Autodesk Inventor part; units mm, degrees
ref_plane "YZ Plane" through (0, 0, 0) normal (1, 0, 0) x (0, 1, 0)
ref_plane "XZ Plane" through (0, 0, 0) normal (0, 1, 0) x (-1, 0, 0)
ref_plane "XY Plane" through (0, 0, 0) normal (0, 0, 1) x (1, 0, 0)
sketch "Sketch1" plane through (0, 0, 0) normal (0, 0, 1) x (1, 0, 0)
  line L0 (-22, 35) -> (22, 35)
  line L1 (22, 35) -> (22, -35)
  line L2 (22, -35) -> (-22, -35)
  line L3 (-25, -38) -> (25, -38)
  line L4 (25, -38) -> (25, 38)
  line L5 (25, 38) -> (-25, 38)
  line L6 (-25, 38) -> (-25, -38)
  line L7 (-22, -6.5359) -> (-22, 6.5359)
  arc A0 (-22, -6.5359) -> (-22, -13.4641) centre (-20, -10) ccw
  arc A1 (-22, 13.4641) -> (-22, 6.5359) centre (-20, 10) ccw
  line L8 (-22, 13.4641) -> (-22, 35)
  line L9 (-22, -35) -> (-22, -13.4641)
  point P0 (0, 0)
extrude "Extrusion1" add sketch "Sketch1" along normal blind 2 contours L0 L1 L2 L9 A0 L7 A1 L8 | L6 L5 L4 L3
sketch "Sketch2" plane through (-25, -38, 0) normal (0, -1, 0) x (1, 0, 0)
  line L0 (50, 0) -> (103.092, -17) construction
  line L1 (43.7539, 2) -> (50, 0)
  line L2 (0, 2) -> (50, 2) construction
  line L3 (50, 0) -> (50, 2)
  line L4 (43.7539, 2) -> (50, 2)
  line L5 (50, 2) -> (50, 0)
  point P0 (25, 0)
extrude "Extrusion2" cut sketch "Sketch2" against normal through all
sketch "Sketch3" plane through (0, 0, 0) normal (0, 0, -1) x (-1, 0, 0)
  line L0 (-22, -35) -> (22, -35)
  line L1 (22, 35) -> (-22, 35)
  line L2 (-22, 35) -> (-22, -35)
  line L3 (22, -35) -> (22, -13.4641)
  line L4 (22, 13.4641) -> (22, 35)
  line L5 (-21.5, -34.5) -> (21.5, -34.5)
  line L6 (21.5, -34.5) -> (21.5, -32.5)
  line L7 (21.5, -32.5) -> (-21.5, -32.5)
  line L8 (-21.5, -32.5) -> (-21.5, -34.5)
  line L9 (-21.5, 32.5) -> (21.5, 32.5)
  line L10 (21.5, 32.5) -> (21.5, 34.5)
  line L11 (21.5, 34.5) -> (-21.5, 34.5)
  line L12 (-21.5, 34.5) -> (-21.5, 32.5)
  point P0 (0, 0)
  dimension "d4" = 0.5
  dimension "d5" = 0.5
  dimension "d6" = 0.5
  dimension "d8" = 0.5
  dimension "d9" = 2
  dimension "d10" = 2
extrude "Extrusion3" add sketch "Sketch3" along normal blind 10
equation "\"d5\" = d4"
equation "\"d6\" = d4"
equation "\"d8\" = d4"
equation "\"d10\" = d9"
properties part number "cover2" material "Ogólne"
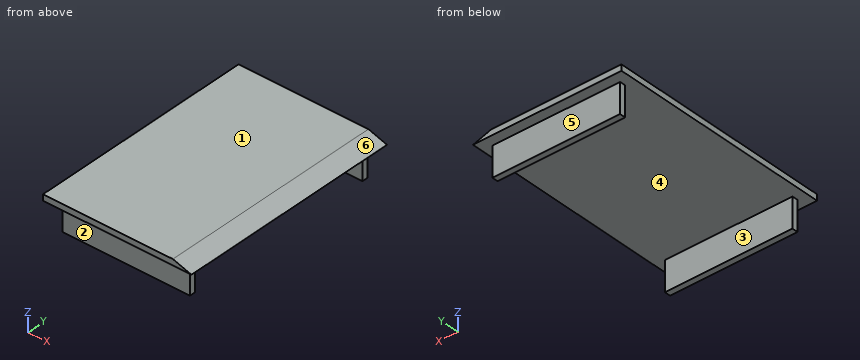
Geometry check sheet. Reference: the model listing, model coordinates, mm. Face numbers are marked on the shaded views. A direction names the side the tool comes from. Give positions to 0.01 mm unless a question says otherwise; leave off trailing zeros. Loops run counter-clockwise (first coordinate to the right, second up) from the corner with the lowest first, then second, coordinate; pieces in that order, holes last. Notation, with made-up numbers: (-12, -32.5) -> (23, -32.5) arc R26 ccw to (23, -15.5) -> close; hole circle Ø3 at (76.25, -4). An arc over 180 degrees is marked (long way). Answer in a Markdown table with one row per item. Add a question column.
1) Cross-section at D-D on x = 20. Record the boundary of the cut face in (y, z), and give its area (3 significant figures).
2) Set-up check for the marked faces 1, 2 and 3: record each of +Z, -Z, +X, -X, +Y, -Y from which the full face is reachable in a straight line by a thin tool's end or side.
3) Cross-section at A-A on z = -6.5. Record the boundary of the cut face in (x, y).
4) Draft check along Y on the marked faces 4, 5 and 6. Enter one of: pulls with the +Y half, pulls with the -Y half, needs draft (parallel to the pull), parting line crosses it, or undercut.
5) Cross-section at B-B on x = -19.5. Record the boundary of the cut face in (y, z), and give its area (3 significant figures).
6) Gauge pin test, flat ends, axial feed: P1, Ø1.6, axis at y = 33.5, z = -3, coming from the +X side; P2, Ø5, axis at x = 3.5, z = -4.5, coming from the +Y side; P3, Ø1.5, axis at x = -17.5, z = -6.5, coming from the -Y side. Record the tip position at first contact, or that the pin passes through.
7) Material ranges on probe 1 along Y at (x, z) = (-19, -8); probe 2 along Z at (x, y) = (-13, -9); probe 3 along Z at (x, y) = (20, -5.5), recorded low to high. Write a range as from..to.
8) Cross-section at C-C on y = 11.5. Record the boundary of the cut face in (x, z).
Outcome:
| question | item | result |
|---|---|---|
| 1 | outline | (-38, 0) -> (-34.5, 0) -> (-34.5, -10) -> (-32.5, -10) -> (-32.5, 0) -> (32.5, 0) -> (32.5, -10) -> (34.5, -10) -> (34.5, 0) -> (38, 0) -> (38, 1.6) -> (-38, 1.6) -> close |
| 1 | area | 162 mm^2 |
| 2 | face 1 | +Z, +X, -X, +Y, -Y |
| 2 | face 2 | -Z, +X, -X, -Y |
| 2 | face 3 | -Z, +X, -X |
| 3 | outline | (-21.5, -34.5) -> (21.5, -34.5) -> (21.5, -32.5) -> (-21.5, -32.5) -> close; (-21.5, 32.5) -> (21.5, 32.5) -> (21.5, 34.5) -> (-21.5, 34.5) -> close |
| 4 | face 4 | undercut |
| 4 | face 5 | pulls with the +Y half |
| 4 | face 6 | needs draft |
| 5 | outline | (-38, 0) -> (-34.5, 0) -> (-34.5, -10) -> (-32.5, -10) -> (-32.5, 0) -> (32.5, 0) -> (32.5, -10) -> (34.5, -10) -> (34.5, 0) -> (38, 0) -> (38, 2) -> (-38, 2) -> close |
| 5 | area | 192 mm^2 |
| 6 | P1 | stops at x = 21.5 |
| 6 | P2 | stops at y = 34.5 |
| 6 | P3 | stops at y = -34.5 |
| 7 | probe 1 | y = -34.5..-32.5, 32.5..34.5 |
| 7 | probe 2 | z = 0..2 |
| 7 | probe 3 | z = 0..1.6 |
| 8 | outline | (-25, 0) -> (25, 0) -> (18.75, 2) -> (-25, 2) -> close |
